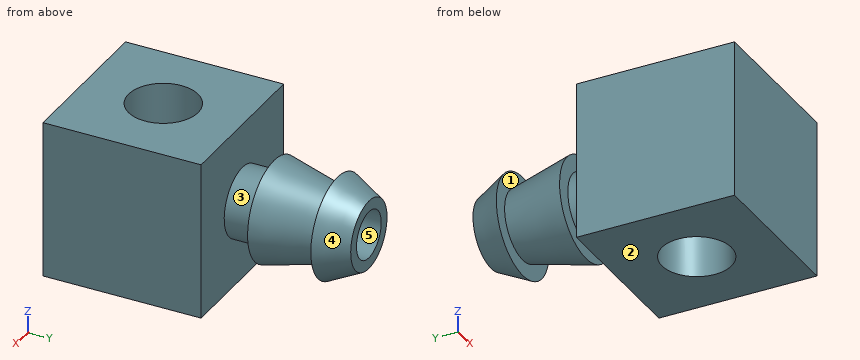
from build123d import *

# Parameters (mm, degrees)
SKETCH1_W           = 5
SKETCH1_H           = 5
BOSS_EXTRUDE1_DEPTH = 5
SKETCH5_R           = 0.75
CUT_EXTRUDE1_DEPTH  = 8
SKETCH6_R           = 1.1
CUT_EXTRUDE2_DEPTH  = 8


with BuildPart() as part:
    # Sketch1 → Boss-Extrude1 (new body)
    with BuildSketch(Plane.XY):
        Rectangle(SKETCH1_W, SKETCH1_H)
    extrude(amount=BOSS_EXTRUDE1_DEPTH)

    # Sketch2 → Revolve1 (revolve)
    with BuildSketch(Plane(origin=(0, 0, 0), x_dir=(0, 0, -1), z_dir=(1, 0, 0))):
        Polygon((-2.5, 2.5), (-2.5, 6.5), (-3.6, 6.5), (-4.1, 5.5), (-3.6, 5.5), (-4.1, 3.5), (-3.6, 3.5), (-3.6, 2.5), align=None)
    revolve(axis=Axis((0, 2.5, 2.5), (0, 1, 0)))

    # Sketch5 → Cut-Extrude1 (cut)
    with BuildSketch(Plane(origin=(0, 6.5, 0), x_dir=(1, 0, 0), z_dir=(0, 1, 0))):
        with Locations((0, -2.5)):
            Circle(SKETCH5_R)
    extrude(amount=-CUT_EXTRUDE1_DEPTH, mode=Mode.SUBTRACT)

    # Sketch6 → Cut-Extrude2 (cut)
    with BuildSketch(Plane(origin=(0, 0, 0), x_dir=(-1, 0, 0), z_dir=(0, 0, -1))):
        Circle(SKETCH6_R)
    extrude(amount=-CUT_EXTRUDE2_DEPTH, mode=Mode.SUBTRACT)


solid = part.part
Check sheet for the modelled part. Datum: model origin and axes. Units: mm. Face numbers are marked on the shaded views. A direction names the side the tool comes from. Round coordinates to 2 decimals unless told otherwise and drop trailing zeros. Loops run counter-clockwise (first coordinate to the right, second up) from the corner with the lowest first, then second, coordinate; pieces in that order, holes last. Notation, with made-up numbers: (63, -17) -> (119, -17) arc R18 cw to (119, 0) -> close; hole circle Ø5 at (23.5, 89.25). An arc over 180 degrees is marked (long way). Put each result on its own line as item: value. Start each with the question number.
1. Section check C-C (z = 4.2). Enter the section's corners in (x, y), plus the area to 3 significant figures.
2. Access from +Z, -Z, +X, -X, +Y, -Y to the whole of each face (thin tool, end or side, straight path). Record for the marked faces 1 and 2.
3. Draft check along Y on the marked faces 3, 4 and 5. Enter one of: +Y half, -Y half, draft (parallel to the pull), parting line (faces both ways), or undercut.
4. Section check B-B (x = 0). Enter the section's corners in (y, z), plus the area to 3 significant figures.
5. Section check D-D (z = 2.5). Enter the section's corners in (x, y).
6. Scan lines: probe 1 along X at (y, z) = (3.25, 2.5); probe 2 along Z at (x, y) = (0, -1.2); probe 3 along X at (y, z) = (-1.1, 2.5). Record each from-to range of solid material in increasing order.
7. Section check A-A (y = 0). Enter the section's corners in (x, z), plus the area to 3 significant figures.
8. Gauge pin test, flat ends, axial feed: pin 1 (3 mm diameter, centred on x = -2, y = 5, fed in from -Z); pin 2 (1.2 mm diameter, centred on x = 0, z = 2.5, fed in from +Y). Record the tip position at first contact, or that the pin passes through.
Findings:
1. outline: (-2.5, -2.5) -> (2.5, -2.5) -> (2.5, 2.5) -> (-2.5, 2.5) -> close; hole circle Ø2.2 at (0, 0)
1. area: 21.2 mm^2
2. face 1: none
2. face 2: -Z, +X, -X, +Y, -Y
3. face 3: undercut
3. face 4: +Y half
3. face 5: draft
4. outline: (-2.5, 0) -> (-1.1, 0) -> (-1.1, 1.75) -> (-1.5, 1.75) -> (-1.5, 3.25) -> (-1.1, 3.25) -> (-1.1, 5) -> (-2.5, 5) -> close; (1.1, 0) -> (2.5, 0) -> (2.5, 1.4) -> (3.5, 1.4) -> (3.5, 0.9) -> (5.5, 1.4) -> (5.5, 0.9) -> (6.5, 1.4) -> (6.5, 1.75) -> (1.1, 1.75) -> close; (1.1, 3.25) -> (6.5, 3.25) -> (6.5, 3.6) -> (5.5, 4.1) -> (5.5, 3.6) -> (3.5, 4.1) -> (3.5, 3.6) -> (2.5, 3.6) -> (2.5, 5) -> (1.1, 5) -> close
4. area: 15.6 mm^2
5. outline: (-2.5, -2.5) -> (2.5, -2.5) -> (2.5, 2.5) -> (1.1, 2.5) -> (1.1, 3.5) -> (1.6, 3.5) -> (1.1, 5.5) -> (1.6, 5.5) -> (1.1, 6.5) -> (0.75, 6.5) -> (0.75, 0.8) arc R1.1 cw to (0.75, -0.8) -> (0.75, -1.5) -> (-0.75, -1.5) -> (-0.75, -0.8) arc R1.1 cw to (-0.75, 0.8) -> (-0.75, 6.5) -> (-1.1, 6.5) -> (-1.6, 5.5) -> (-1.1, 5.5) -> (-1.6, 3.5) -> (-1.1, 3.5) -> (-1.1, 2.5) -> (-2.5, 2.5) -> close
6. probe 1: x = -1.1 to -0.75, 0.75 to 1.1
6. probe 2: z = 0 to 1.75, 3.25 to 5
6. probe 3: x = -2.5 to -0.75, 0.75 to 2.5
7. outline: (-2.5, 0) -> (-1.1, 0) -> (-1.1, 5) -> (-2.5, 5) -> close; (1.1, 0) -> (2.5, 0) -> (2.5, 5) -> (1.1, 5) -> close
7. area: 14.0 mm^2
8. pin 1: stops at z = 1.01
8. pin 2: stops at y = -1.5
